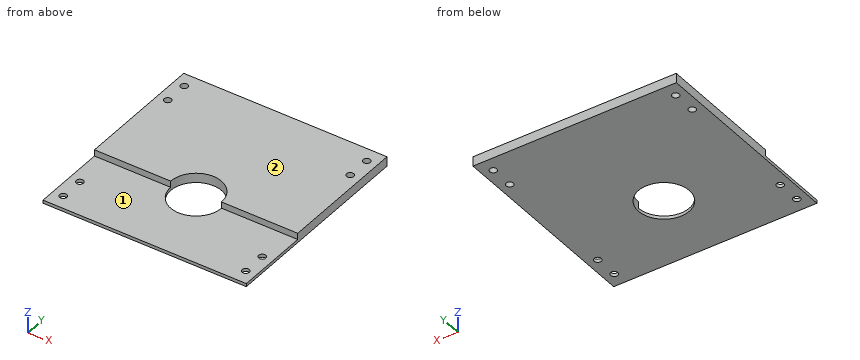
```python
from build123d import *

# Parameters (mm, degrees)
SKETCH_1_W          = 406.4
SKETCH_1_H          = 406.4
SKETCH_1_R          = 50.8
EXTRUDE_1_DEPTH     = 19.05
CUT_EXTRUDE_START   = -12.7
CUT_EXTRUDE_1_DEPTH = 12.7
SKETCH_4_R          = 7.112
CUT_EXTRUDE_4_DEPTH = 288.998927949


with BuildPart() as part:
    # 草图1 → 凸台-拉伸1 (new body)
    with BuildSketch(Plane.XY):
        Rectangle(SKETCH_1_W, SKETCH_1_H)
        with Locations(Location((0, -54.602000016, 0), (0, 0, 180))):
            Circle(SKETCH_1_R, mode=Mode.SUBTRACT)
    extrude(amount=EXTRUDE_1_DEPTH)

    # 草图3 → 切除-拉伸1 (cut)
    with BuildSketch(Plane.XY.offset(19.05).offset(CUT_EXTRUDE_START)):
        with BuildLine():
            Line((-50.8, -54.602000016), (-203.2, -54.602000016))
            Line((-203.2, -54.602000016), (-203.2, -203.2))
            Line((-203.2, -203.2), (203.2, -203.2))
            Line((203.2, -203.2), (203.2, -54.602000016))
            Line((203.2, -54.602000016), (50.8, -54.602000016))
            ThreePointArc((50.8, -54.602000016), (0, -105.402000016), (-50.8, -54.602000016))
        make_face()
    extrude(amount=CUT_EXTRUDE_1_DEPTH, mode=Mode.SUBTRACT)

    # 草图4 → 切除-拉伸4 (cut, through all)
    with BuildSketch(Plane.XY):
        with Locations(Location((-182.372, 174.752, 0), (0, 0, 180))):
            Circle(SKETCH_4_R)
        with Locations(Location((-182.372, 127, 0), (0, 0, 180))):
            Circle(SKETCH_4_R)
        with Locations(Location((182.372, 127, 0), (0, 0, 180))):
            Circle(SKETCH_4_R)
        with Locations(Location((182.372, 174.752, 0), (0, 0, 180))):
            Circle(SKETCH_4_R)
        with Locations(Location((182.372, -174.752, 0), (0, 0, 180))):
            Circle(SKETCH_4_R)
        with Locations(Location((182.372, -127, 0), (0, 0, 180))):
            Circle(SKETCH_4_R)
        with Locations(Location((-182.372, -174.752, 0), (0, 0, 180))):
            Circle(SKETCH_4_R)
        with Locations(Location((-182.372, -127, 0), (0, 0, 180))):
            Circle(SKETCH_4_R)
    extrude(amount=CUT_EXTRUDE_4_DEPTH, mode=Mode.SUBTRACT)


solid = part.part
```
Geometry: final body of the model. Coordinates: model frame, mm. Face numbers are marked on the shaded views. A direction names the side the tool comes from. Coordinates: 2 decimals unless noted, no trailing zeros. Order: outer loops, then holes, each group sorted by start corner. A loop starts at its lowest first (then second) coordinate and runs counter-clockwise, first axis right, second up. Notation, with made-up numbers: M 24.25,60.5 L 28.25,60.5 A34 cw 28.25,93.5 Z; hole C -38,82 d7. An arc over 180 degrees is marked long. Answer in a Markdown table with one row per item. Add a question column.
Q1. Contact query for flat-ended pins moving along their axis: P1, Ø2, axis at x = -107, z = 10.5, coming from the -Y side; P2, Ø13, axis at x = 182.372, y = 127, coming from the +Z side. Output: stop coordinate, or through.
Q2. Section query B-B on x = 0. Return the cut outline in (y, z), and give its area (3 significant figures).
Q3. Section query C-C on y = -127. Return the cut outline in (x, z).
Q4. Section query A-A on y = 127. Return the cut outline in (x, z).
Q5. Line query: L1, parallel to X at y = 127, z = 6.25; L2, parallel to X at y = -57.5, z = 1.5; L3, parallel to Y at x = 0, z = 6. Output: solid intervals per line, ascending.
Q6. Section query D-D on z = 10.25. Return the cut outline in (x, y), and give its area (3 significant figures).
Q7. Reachability of the marked faces 1 and 2 from +Z, -Z, +X, -X, +Y, -Y: full face, straight path, thin tool, end or side. Return the list, or none.
Completed:
| question | item | result |
|---|---|---|
| 1 | P1 | stops at y = -54.6 |
| 1 | P2 | passes through |
| 2 | outline | M -203.2,0 L -105.4,0 L -105.4,6.35 L -203.2,6.35 Z; M -3.8,0 L 203.2,0 L 203.2,19.05 L -3.8,19.05 Z |
| 2 | area | 4,560 mm2 |
| 3 | outline | M -203.2,0 L -189.48,0 L -189.48,6.35 L -203.2,6.35 Z; M -175.26,0 L 175.26,0 L 175.26,6.35 L -175.26,6.35 Z; M 189.48,0 L 203.2,0 L 203.2,6.35 L 189.48,6.35 Z |
| 4 | outline | M -203.2,0 L -189.48,0 L -189.48,19.05 L -203.2,19.05 Z; M -175.26,0 L 175.26,0 L 175.26,19.05 L -175.26,19.05 Z; M 189.48,0 L 203.2,0 L 203.2,19.05 L 189.48,19.05 Z |
| 5 | L1 | x = -203.2 to -189.48, -175.26 to 175.26, 189.48 to 203.2 |
| 5 | L2 | x = -203.2 to -50.72, 50.72 to 203.2 |
| 5 | L3 | y = -203.2 to -105.4, -3.8 to 203.2 |
| 6 | outline | M -203.2,-54.6 L -50.8,-54.6 A50.8 cw 50.8,-54.6 L 203.2,-54.6 L 203.2,203.2 L -203.2,203.2 Z; hole C -182.37,127 d14.22; hole C -182.37,174.75 d14.22; hole C 182.37,127 d14.22; hole C 182.37,174.75 d14.22 |
| 6 | area | 100,000 mm2 |
| 7 | face 1 | +Z, +X, -X, -Y |
| 7 | face 2 | +Z, +X, -X, +Y, -Y |
